Geometry check sheet. Reference: drawing and pictorial views, mm from the part's lowest x, y, z. Round coordinates to 2 decimals unless told otherwise and drop trailing zeros. Order: outer loops, then holes, each group sorted by start corner. A loop starts at its lowest first (then second) coordinate and runs counter-clockwise, first axis right, second up.
(1) Sectioned sample at B-B, the plane x = 5. Enter the section's corners in (y, z).
(2) Thickness scan on probe 1 along Y at (x, z) = (5, 1.4). Record the ranges inside material, lowest first.
(3) Depth check by flat-ended pin: pin 1 (1.6 mm diameter, centred on x = 37, y = 21, fed in from +Z). Enter the tip coordinate at first touch or a pass-through.
(4) Sectioned sample at A-A, the plane y = 2. Enter the section's corners in (x, z), and give its area (3 significant figures).
(5) Mould release check, pull along Y, two halves, no side actions. Record for the marked faces 1 and 2: released by +Y, released by -Y, zero draft, split by the parting line, or undercut.
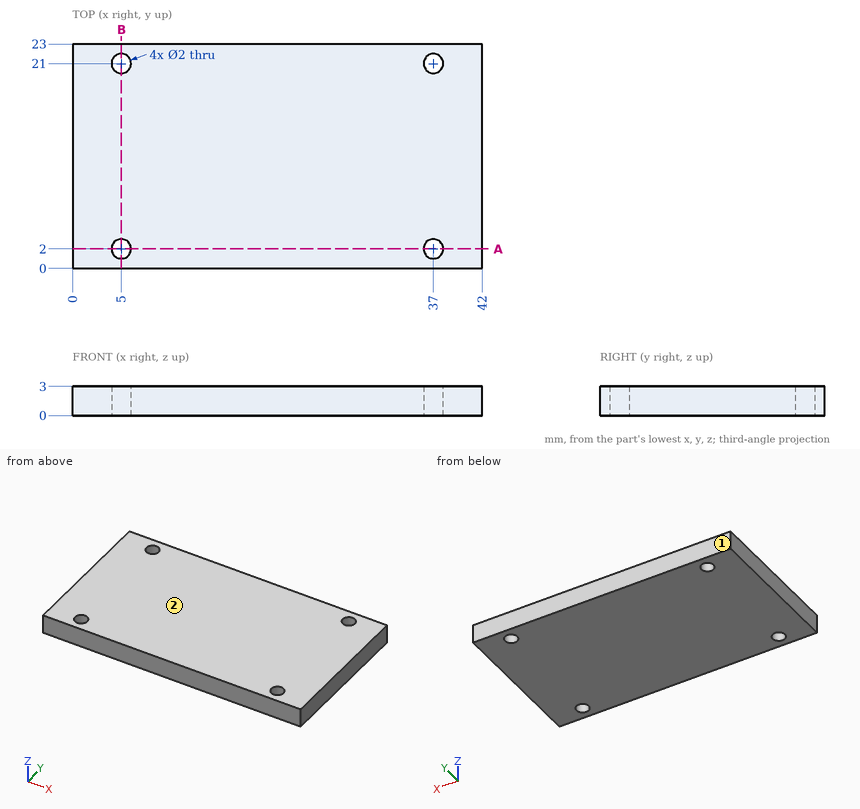
Derived:
1. outline: (0, 0) - (1, 0) - (1, 3) - (0, 3) - close; (3, 0) - (20, 0) - (20, 3) - (3, 3) - close; (22, 0) - (23, 0) - (23, 3) - (22, 3) - close
2. probe 1: y = 0 to 1, 3 to 20, 22 to 23
3. pin 1: passes through
4. outline: (0, 0) - (4, 0) - (4, 3) - (0, 3) - close; (6, 0) - (36, 0) - (36, 3) - (6, 3) - close; (38, 0) - (42, 0) - (42, 3) - (38, 3) - close
4. area: 114 mm2
5. face 1: released by +Y
5. face 2: zero draft
